Could you check a few things on this drawing? It's one solid part, dimensions in mm from its lowest x, y, z. A direction names the side the tool comes from. Coordinates: 2 decimals unless noted, no trailing zeros. Write each loop counter-clockwise with the first axis right and the second up, starting at its lowest first coordinate (ties: lowest second). Pieces come first, ordered by that corner, then holes. Notation, with made-up numbers: (88, 21.5) - (142, 21.5) arc R15 cw to (142, 42.5) - close; hole circle Ø2 at (34, 19). An arc over 180 degrees is marked (long way). Answer as a JSON object with one key per item and string values. Group by question number.
1) We'd pull the mould along X, two halves only. Please class the marked faces 3, 4, 5 and 6: released by +X, released by -X, zero draft, split by the parting line, or undercut.
2) If we section it at B-B (z = 17): Write out the boundary of the cut face in (x, y).
3) If we section it at A-A (x = 30): Write out the boundary of the cut face in (y, z), plus the area to 3 significant figures.
4) Will these pins go through, and if not, where does the flat tip stop? pin 1 Ø1 at (x, y) = (10, 4.5) entering from -Z; pin 2 Ø3 at (y, z) = (8.5, 3) entering from -X; pin 3 Ø5 at (x, y) = (30, 10) entering from -Z.
5) If we section it at D-D (y = 10): Write out the boundary of the cut face in (x, z), plus the area to 3 significant figures.
6) If we section it at C-C (x = 5): Write out the boundary of the cut face in (y, z).
7) On a 3-axis mill with a long thin cutter (end or side, diameter ignored), from which of +Z, -Z, +X, -X, +Y, -Y can I reach the whole of each face in a straight line? I mean the marked faces 1 and 2. Say none if no direction works.
8) Please list where these lines run through material, in increasing order: line 1 along Y through (x, z) = (5, 20); line 2 along Y through (x, z) = (30, 6); line 3 along Z through (x, y) = (14, 9.5).
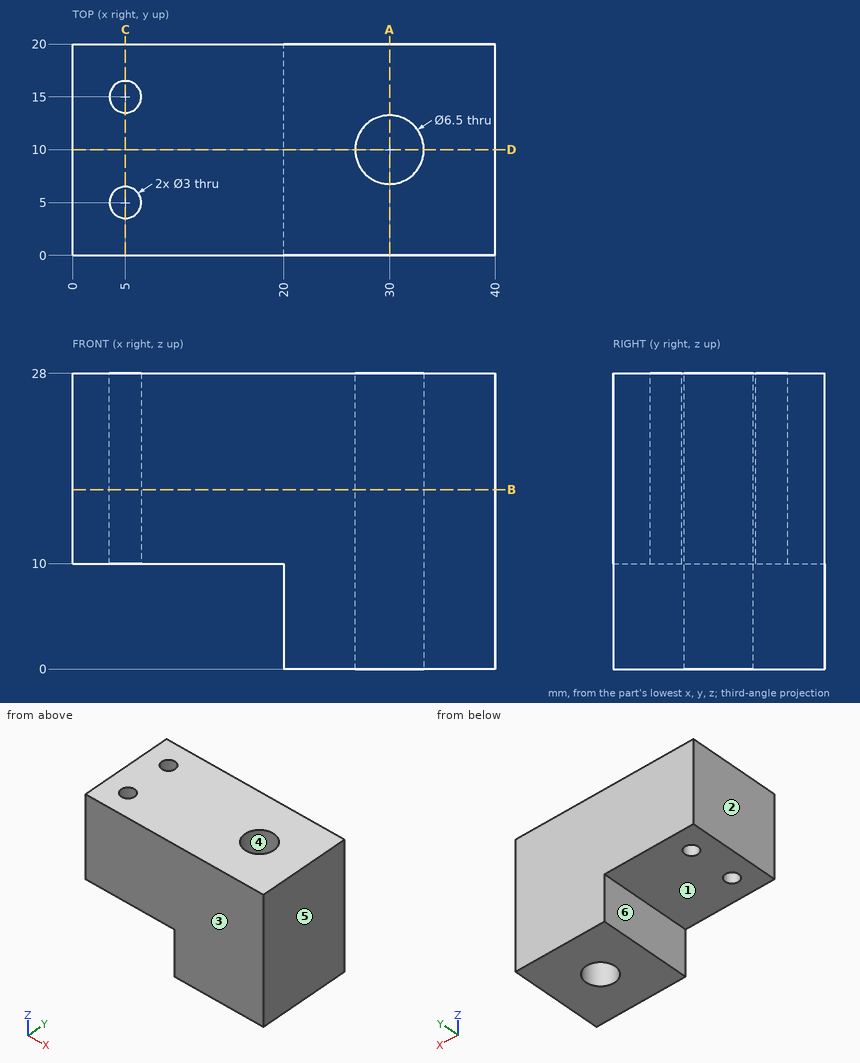
Here are the results:
{
 "1": {"face 3": "zero draft", "face 4": "undercut", "face 5": "released by +X", "face 6": "released by -X"},
 "2": {"outline": "(0, 0) - (40, 0) - (40, 20) - (0, 20) - close; hole circle Ø3 at (5, 5); hole circle Ø3 at (5, 15); hole circle Ø6.5 at (30, 10)"},
 "3": {"outline": "(0, 0) - (6.75, 0) - (6.75, 28) - (0, 28) - close; (13.25, 0) - (20, 0) - (20, 28) - (13.25, 28) - close", "area": "378 mm²"},
 "4": {"pin 1": "stops at z = 10", "pin 2": "stops at x = 20", "pin 3": "passes through"},
 "5": {"outline": "(0, 10) - (20, 10) - (20, 0) - (26.75, 0) - (26.75, 28) - (0, 28) - close; (33.25, 0) - (40, 0) - (40, 28) - (33.25, 28) - close", "area": "738 mm²"},
 "6": {"outline": "(0, 10) - (3.5, 10) - (3.5, 28) - (0, 28) - close; (6.5, 10) - (13.5, 10) - (13.5, 28) - (6.5, 28) - close; (16.5, 10) - (20, 10) - (20, 28) - (16.5, 28) - close"},
 "7": {"face 1": "-Z, -X, +Y, -Y", "face 2": "+Z, -Z, -X, +Y, -Y"},
 "8": {"line 1": "y = 0 to 3.5, 6.5 to 13.5, 16.5 to 20", "line 2": "y = 0 to 6.75, 13.25 to 20", "line 3": "z = 10 to 28"}
}
